For this review, take the finished solid that the model builds, in its own axes (mm). Face numbers are marked on the shaded views. A direction names the side the tool comes from. Coordinates: 2 decimals unless noted, no trailing zeros. Write each loop counter-clockwise with the first axis right and the second up, starting at its lowest first coordinate (ties: lowest second). Pieces come first, ordered by that corner, then holes.
```python
from build123d import *

# Parameters (mm, degrees)
F2_R     = 800
F2_R_2   = 120
F3_DEPTH = 25
F4_W     = 80
F4_H     = 70
F5_DEPTH = 395.001


with BuildPart() as f1:
    # F0 (on Front) → F1 (revolve)
    with BuildSketch(Plane.XZ):
        with BuildLine():
            Line((120, 370), (120, 0))
            Line((120, 0), (270, 0))
            Line((270, 0), (270, 83.724369))
            Line((270, 83.724369), (200, 83.724369))
            Line((200, 83.724369), (200, 233.724369))
            Line((200, 233.724369), (270, 233.724369))
            Line((270, 233.724369), (270, 313.724369))
            Line((270, 313.724369), (952.792001, 313.724369))
            Line((952.792001, 313.724369), (952.792001, 382.131195))
            Line((952.792001, 382.131195), (900, 720))
            Line((900, 720), (850, 720))
            Line((850, 720), (850, 420))
            ThreePointArc((850, 420), (835.355339, 384.644661), (800, 370))
            Line((800, 370), (120, 370))
        make_face()
    revolve(axis=Axis((0, 0, -17.114428), (0, 0, -1)))

    # F2 (on face) → F3 (join)
    with BuildSketch(Plane.XY.offset(370)):
        Circle(F2_R)
        Circle(F2_R_2, mode=Mode.SUBTRACT)
    extrude(amount=F3_DEPTH)

    # F4 (on face) → F5 (cut, through all)
    with BuildSketch(Plane.XY.offset(395)):
        with Locations((0, 120)):
            Rectangle(F4_W, F4_H)
    extrude(amount=-F5_DEPTH, mode=Mode.SUBTRACT)


solid = f1.part
```
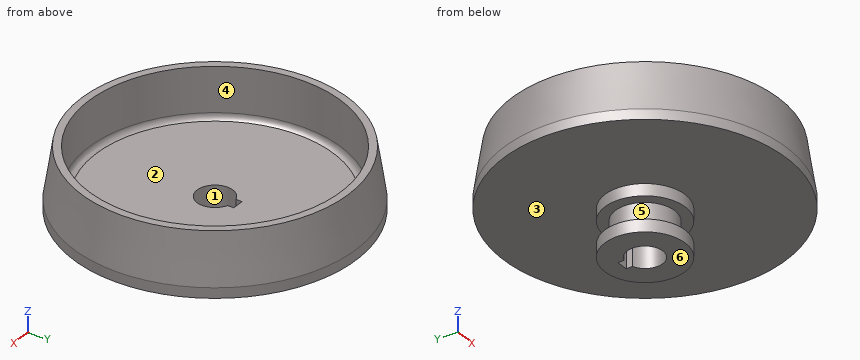
Q1. For probe 1 along Y at (x, z) = (0, 103); probe 2 along X at (y, z) = (0, 225); probe 3 along Z at (x, y) = (219, -82.5), list the stretches that pass through material, from the lowest coordinate up.
Ans:
probe 1: y = -200 to -120, 155 to 200
probe 2: x = -200 to -120, 120 to 200
probe 3: z = 0 to 83.72, 233.72 to 395
Q2. Clearance check with flat-ended pins moving along their axes: pin 1 Ø1.5 at (x, z) = (-614, 416) entering from +Y; pin 2 Ø3 at (x, y) = (-17, -494) entering from -Z; pin 3 Ø1 at (x, z) = (227.5, 417.5) entering from +Y. State where each tip first meets the part, or that it passes through.
Ans:
pin 1: stops at y = 722.29
pin 2: stops at z = 313.72
pin 3: stops at y = 919.69
Q3. Tool access review of the marked faces 1, 2 and 3: name each direction out of +Z, -Z, +X, -X, +Y, -Y from which nothing blocks a thin tool from reaching the whole face with its end or side.
Ans:
face 1: +Z, -Z
face 2: +Z
face 3: -Z
Q4. Draft analysis for pull direction X (two halves, no side actions). For the marked faces 4, 5 and 6, state which applies: +X half, -X half, draft (parallel to the pull), parting line (faces both ways), or undercut.
Ans:
face 4: undercut
face 5: parting line
face 6: draft
Q5. Add section C-C (z = 541.5). State the section outline as (x, y) points.
Ans:
outline: circle Ø1855.78 at (0, 0); hole circle Ø1700 at (0, 0)
